Verification items for this drawing (mm, ordinates from the low corner). A direction names the side the tool comes from. Round coordinates to 2 decimals unless told otherwise and drop trailing zeros. Write each loop counter-clockwise with the first axis right and the second up, starting at its lowest first coordinate (ties: lowest second). Pieces come first, ordered by that corner, then holes. Notation, with made-up numbers: M 64,70 L 83,70 A25 ccw 83,103 Z; hole C 34.5,8.25 d5. An arc over 180 degrees is marked long. Write each question's results on one line, items separated by ' | '.
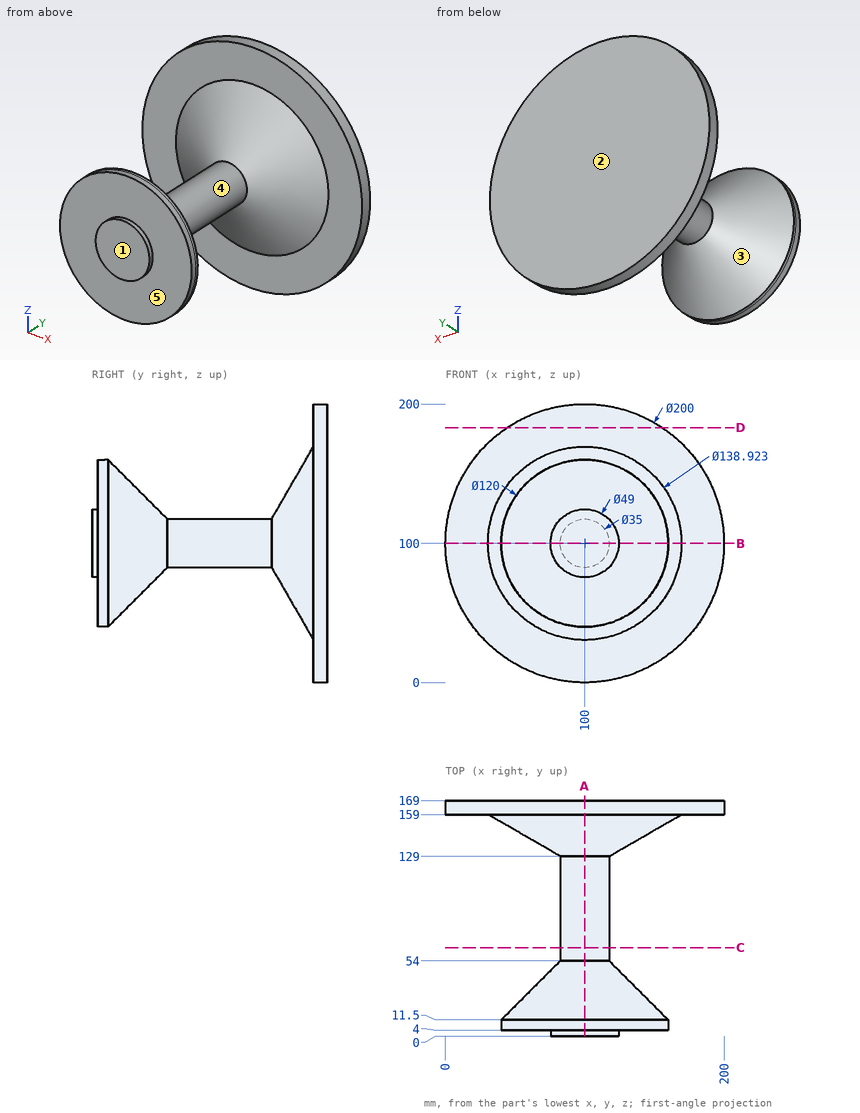
1) Depth check by flat-ended pin: P1, Ø4, axis at x = 177, z = 112, coming from the -Y side; P2, Ø1.5, axis at x = 46.5, z = 69.5, coming from the -Y side; P3, Ø5, axis at y = 71, z = 92.5, coming from the +X side. Enter the tip coordinate at first touch or a pass-through.
Calculated:
P1: stops at y = 159 | P2: stops at y = 154.02 | P3: stops at x = 116.77
2) Sectioned sample at A-A, the plane x = 100. Record the cut outline in (y, z), and give its area (3 significant figures).
Calculated:
outline: M 0,75.5 L 4,75.5 L 4,40 L 11.5,40 L 54,82.5 L 129,82.5 L 159,30.54 L 159,0 L 169,0 L 169,200 L 159,200 L 159,169.46 L 129,117.5 L 54,117.5 L 11.5,160 L 4,160 L 4,124.5 L 0,124.5 Z | area: 11,600 mm²
3) Sectioned sample at D-D, the plane z = 183. Record the cut outline in (x, y).
Calculated:
outline: M 44.22,159 L 155.78,159 L 155.78,169 L 44.22,169 Z
4) Access from +Z, -Z, +X, -X, +Y, -Y to the whole of each face (thin tool, end or side, straight path). Record for the marked faces 4 and 5.
Calculated:
face 4: none | face 5: -Y
5) Sectioned sample at C-C, the plane y = 63.5. Record the cut outline in (x, z).
Calculated:
outline: C 100,100 d35
6) Draft check along Y on the marked faces 1, 2 and 3. Enter one of: pulls with the +Y half, pulls with the -Y half, needs draft (parallel to the pull), parting line crosses it, or undercut.
Calculated:
face 1: pulls with the -Y half | face 2: pulls with the +Y half | face 3: undercut
7) Sectioned sample at B-B, the plane z = 100. Record the cut outline in (x, y).
Calculated:
outline: M 0,159 L 30.54,159 L 82.5,129 L 82.5,54 L 40,11.5 L 40,4 L 75.5,4 L 75.5,0 L 124.5,0 L 124.5,4 L 160,4 L 160,11.5 L 117.5,54 L 117.5,129 L 169.46,159 L 200,159 L 200,169 L 0,169 Z
8) Material ranges on line 1 (Y direction, x = 131.5, z = 11); line 2 (Y direction, x = 65, z = 104) (3 decimals); line 3 (Y direction, x = 91, z = 52.5) (1 decimal), recorded low to high. Write a range as [from, to].
Calculated:
line 1: y = [159, 169] | line 2: y = [4, 36.272], [139.235, 169] | line 3: y = [4, 23.2], [146.8, 169]
